Work out the finished part from the listing and answer in its coordinate system (mm). A direction names the side the tool comes from. Round coordinates to 2 decimals unless told otherwise and drop trailing zeros. Loops run counter-clockwise (first coordinate to the right, second up) from the corner with the lowest first, then second, coordinate; pieces in that order, holes last.
```python
from build123d import *

# Parameters (mm, degrees)
F0_R     = 12.5
F1_DEPTH = 160
F3_DEPTH = 40


# Not quite as in the source:
# - a feature names something its author has since deleted; it is built from what else it names


with BuildPart() as f1:
    # F0 (on Top) → F1 (new body)
    with BuildSketch(Plane.XY):
        Circle(F0_R)
    extrude(amount=F1_DEPTH)

    # F2 (on face) → F3 (cut)
    with BuildSketch(Plane.XY.offset(160)):
        with BuildLine():
            ThreePointArc((-2.75, 6.7082039325), (-4.0388736054, -6.0207972894), (7.25, 0))
            ThreePointArc((7.25, 0), (6.0207972894, 4.0388736054), (2.75, 6.7082039325))
            Line((2.75, 6.7082039325), (2.75, 4.75))
            Line((2.75, 4.75), (-2.75, 4.75))
            Line((-2.75, 4.75), (-2.75, 6.7082039325))
        make_face()
        with BuildLine():
            Line((2.75, 4.75), (2.75, 6.7082039325))
            ThreePointArc((2.75, 6.7082039325), (0, 7.25), (-2.75, 6.7082039325))
            Line((-2.75, 6.7082039325), (-2.75, 4.75))
            Line((-2.75, 4.75), (2.75, 4.75))
        make_face()
        with BuildLine():
            ThreePointArc((-2.75, 6.7082039325), (0, 7.25), (2.75, 6.7082039325))
            Line((2.75, 6.7082039325), (2.75, 9.75))
            Line((2.75, 9.75), (-2.75, 9.75))
            Line((-2.75, 9.75), (-2.75, 6.7082039325))
        make_face()
    extrude(amount=-F3_DEPTH, mode=Mode.SUBTRACT)


solid = f1.part
```
1. Consider probe 1 along Y at (x, z) = (0, 137); probe 2 along Z at (x, y) = (1.5, 5); probe 3 along X at (y, z) = (-5.5, 135). Determine where each line is inside the solid, lowest interval first.
Answer key:
probe 1: y = -12.5 to -7.25, 9.75 to 12.5
probe 2: z = 0 to 120
probe 3: x = -11.22 to -4.72, 4.72 to 11.22
2. Find section A-A (z = 149). Write down the section's boundary in (x, y).
Answer key:
outline: circle Ø25 at (0, 0); hole (-2.75, 6.71) arc R7.25 ccw (long way) to (2.75, 6.71) - (2.75, 9.75) - (-2.75, 9.75) - close
3. Find section D-D (z = 100). Write down the section's boundary in (x, y).
Answer key:
outline: circle Ø25 at (0, 0)
4. Given pin 1 (1.5 mm diameter, centred on x = 2.5, z = 53.5, fed in from +Y); pin 2 (8.5 mm diameter, centred on x = 0, y = 0, fed in from +Z); pin 3 (1.5 mm diameter, centred on y = 8.5, z = 135, fed in from +X), each flat-ended and moving along its own axis, determine where each tip first touches the part or whether it passes through.
Answer key:
pin 1: stops at y = 12.38
pin 2: stops at z = 120
pin 3: stops at x = 9.81
5. Find section C-C (y = 5). Write down the section's boundary in (x, z).
Answer key:
outline: (-11.46, 0) - (11.46, 0) - (11.46, 160) - (5.25, 160) - (5.25, 120) - (-5.25, 120) - (-5.25, 160) - (-11.46, 160) - close
6. Which of the six approach directions +Z, -Z, +X, -X, +Y, -Y give full straight-line access (tool end or side, diameter ignored) to faces 4 (the face through (5.4, -5.4, 160)), 5 (the face through (2.75, 8, 140))?
Answer key:
face 4: +Z, +X, -X, +Y, -Y
face 5: +Z
7. Find section B-B (x = 0). Write down the section's boundary in (y, z).
Answer key:
outline: (-12.5, 0) - (12.5, 0) - (12.5, 160) - (9.75, 160) - (9.75, 120) - (-7.25, 120) - (-7.25, 160) - (-12.5, 160) - close
8. Determine the mould class of faces 1 (the face through (0, 0, 0)), 2 (the face through (-2.75, 8, 140)), 3 (the face through (11.923, 3.755, 78.88)) for opening direction X: +X half, -X half, draft (parallel to the pull), parting line (faces both ways), or undercut.
Answer key:
face 1: draft
face 2: undercut
face 3: parting line
